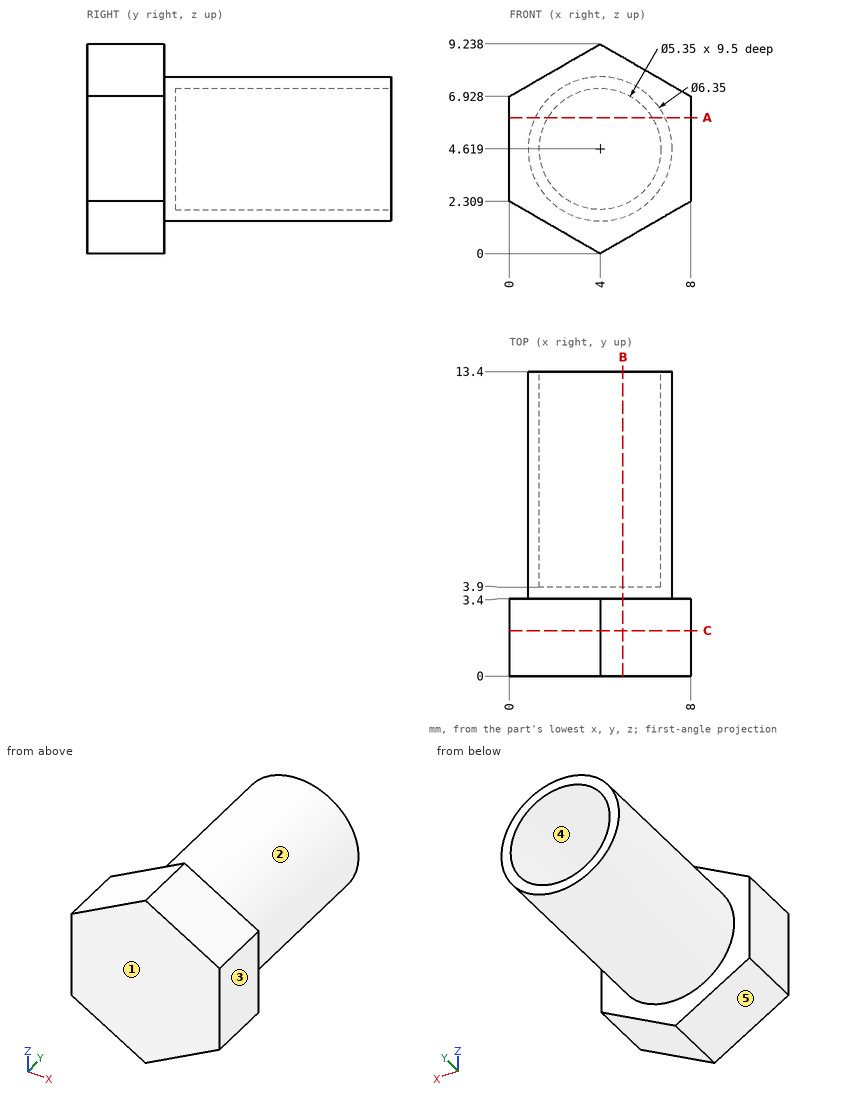
Design review of the part shown in the three views and the two pictorial views. Dimensions are in mm from the part's minimum x, y and z. A direction names the side the tool comes from. Round coordinates to 2 decimals unless told otherwise and drop trailing zeros. Write each loop counter-clockwise with the first axis right and the second up, starting at its lowest first coordinate (ties: lowest second). Pieces come first, ordered by that corner, then holes.
Item 1: Wall thickness on L1, parallel to Z at x = 4, y = 10.5; L2, parallel to Y at x = 5.75, z = 4.75; L3, parallel to Z at x = 3.5, y = 8.75 (1 decimal): over which ranges is each line inside the solid? List them lowest first.
Item 2: Consider section C-C on y = 2. Give the boundary of the cut face in (x, z).
Item 3: For pin 1 Ø1 at (y, z) = (8.5, 5.5) entering from +X; pin 2 Ø3 at (y, z) = (6.5, 7.5) entering from +X; pin 3 Ø1.6 at (x, z) = (3.5, 5.5) entering from +Y, all flat-tipped, find the tip position at first contact; note any pin that passes through.
Item 4: For the marked faces 1 and 2, list the 3-axis set-ups (+Z, -Z, +X, -X, +Y, -Y) from which the entire face can be reached by the end or side of a thin tool; tool diameter is ignored.
Item 5: Consider section B-B on x = 5. Give the boundary of the cut face in (y, z) (1 decimal).
Item 6: Consider section A-A on z = 6. Give the boundary of the cut face in (x, y).
Item 7: Draft analysis for pull direction Z (two halves, no side actions). For the marked faces 3, 4 and 5, state which applies: released by +Z, released by -Z, zero draft, split by the parting line, or undercut.
Check values:
1. L1: z = 1.44 to 1.94, 7.29 to 7.79
1. L2: y = 0 to 3.9
1. L3: z = 1.5 to 2, 7.2 to 7.8
2. outline: (0, 2.31) - (4, 0) - (8, 2.31) - (8, 6.93) - (4, 9.24) - (0, 6.93) - close
3. pin 1: stops at x = 7.15
3. pin 2: stops at x = 6.86
3. pin 3: stops at y = 3.9
4. face 1: +Z, -Z, +X, -X, -Y
4. face 2: +Y
5. outline: (0, 0.6) - (3.4, 0.6) - (3.4, 1.6) - (13.4, 1.6) - (13.4, 2.1) - (3.9, 2.1) - (3.9, 7.1) - (13.4, 7.1) - (13.4, 7.6) - (3.4, 7.6) - (3.4, 8.7) - (0, 8.7) - close
6. outline: (0, 0) - (8, 0) - (8, 3.4) - (6.86, 3.4) - (6.86, 13.4) - (6.29, 13.4) - (6.29, 3.9) - (1.71, 3.9) - (1.71, 13.4) - (1.14, 13.4) - (1.14, 3.4) - (0, 3.4) - close
7. face 3: zero draft
7. face 4: undercut
7. face 5: released by -Z
